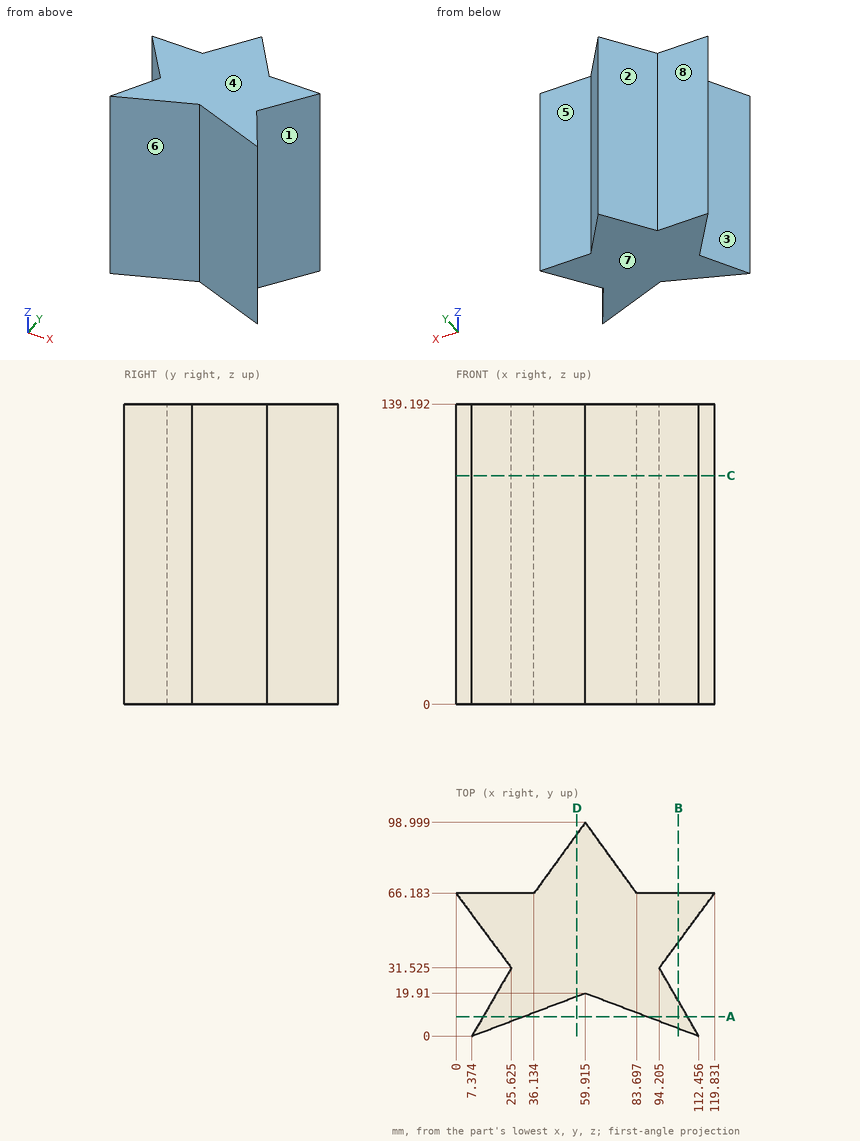
Verification items for this drawing (mm, ordinates from the low corner). A direction names the side the tool comes from. Coordinates: 2 decimals unless noted, no trailing zeros. Order: outer loops, then holes, each group sorted by start corner. A loop starts at its lowest first (then second) coordinate and runs counter-clockwise, first axis right, second up. Notation, with made-up numbers: (-16, 73.5) - (18, 73.5) arc R21 ccw to (18, 78.5) - close; hole circle Ø4 at (56.25, 27.5). An arc over 180 degrees is marked (long way). Answer as a JSON object with one key per item and string values. Group by question number.
Item 1: Scan lines: probe 1 along Y at (x, z) = (109.5, 62.5) (1 decimal); probe 2 along Y at (x, z) = (25.5, 51) (1 decimal); probe 3 along Y at (x, z) = (31, 126). Record each from-to range of solid material in increasing order.
Item 2: Draft check along Y on the marked faces 1, 2, 3 and 4. Enter one of: +Y half, -Y half, draft (parallel to the pull), parting line (faces both ways), or undercut.
Item 3: Sectioned sample at A-A, the plane y = 9. Record the cut outline in (x, z) (1 decimal), and give its area (3 significant figures).
Item 4: Sectioned sample at C-C, the plane z = 106. Record the cut outline in (x, y) (1 decimal).
Item 5: Sectioned sample at D-D, the plane x = 56. Record the cut outline in (y, z), and give its area (3 significant figures).
Item 6: Depth check by flat-ended pin: pin 1 Ø11 at (x, z) = (97, 52.5) entering from +Y; pin 2 Ø2 at (y, z) = (75, 83.5) entering from +X; pin 3 Ø10 at (y, z) = (25, 108.5) entering from +X. Enter the tip coordinate at first touch or a pass-through.
Item 7: Sectioned sample at B-B, the plane x = 103. Record the cut outline in (y, z), and give its area (3 significant figures).
Item 8: Tool access check on the marked faces 5, 6, 7 and 8. Record the directions out of +Z, -Z, +X, -X, +Y, -Y that give a thin tool (end or side, any length) a straight path to the whole face; none if there is none.
Resolved:
{
 "1": {"probe 1": "1.1 to 5.1, 52.2 to 66.2", "probe 2": "6.9 to 31.3, 31.7 to 66.2", "probe 3": "8.95 to 66.18"},
 "2": {"face 1": "undercut", "face 2": "+Y half", "face 3": "undercut", "face 4": "draft"},
 "3": {"outline": "(12.6, 0) - (31.1, 0) - (31.1, 139.2) - (12.6, 139.2) - close; (88.7, 0) - (107.2, 0) - (107.2, 139.2) - (88.7, 139.2) - close", "area": "5,160 mm^2"},
 "4": {"outline": "(0, 66.2) - (25.6, 31.5) - (7.4, 0) - (59.9, 19.9) - (112.5, 0) - (94.2, 31.5) - (119.8, 66.2) - (83.7, 66.2) - (59.9, 99) - (36.1, 66.2) - close"},
 "5": {"outline": "(18.43, 0) - (93.6, 0) - (93.6, 139.19) - (18.43, 139.19) - close", "area": "10,500 mm^2"},
 "6": {"pin 1": "y = 66.18", "pin 2": "x = 78.03", "pin 3": "x = 100.88"},
 "7": {"outline": "(3.58, 0) - (16.33, 0) - (16.33, 139.19) - (3.58, 139.19) - close; (43.42, 0) - (66.18, 0) - (66.18, 139.19) - (43.42, 139.19) - close", "area": "4,940 mm^2"},
 "8": {"face 5": "+Z, -Z, +X, +Y", "face 6": "+Z, -Z, -Y", "face 7": "-Z, +X, -X, +Y, -Y", "face 8": "+Z, -Z, -X, +Y"}
}
